from build123d import *

# Parameters (mm, degrees)
SKETCH1_W                  = 20
SKETCH1_H                  = 13.5
BOSS_EXTRUDE1_DEPTH        = 5
F_3_2_3_2_M2_HEAT_SET_D    = 3.2
FILLET2_R                  = 2.5
F_3_2_3_2_DIAMETER_HOLE1_D = 3.2


with BuildPart() as part:
    # Sketch1 → Boss-Extrude1 (new body)
    with BuildSketch(Plane(origin=(0, 0, 0), x_dir=(1, 0, 0), z_dir=(0, 1, 0))):
        Rectangle(SKETCH1_W, SKETCH1_H)
    extrude(amount=BOSS_EXTRUDE1_DEPTH)

    # Ø3.2 (3.2) M2 heat set (through all)
    with Locations(Plane(origin=(0, 5, 0), x_dir=(1, 0, 0), z_dir=(0, 1, 0))):
        with Locations((0, 3.75)):
            Hole(F_3_2_3_2_M2_HEAT_SET_D / 2)

    # Fillet2
    fillet2_edges = [part.edges().sort_by_distance(p)[0] for p in [
        (0, 0, 6.75),
        (0, 5, 6.75),
    ]]
    fillet(fillet2_edges, radius=FILLET2_R - 0.0001)  # a hair under: the kernel refuses the full size

    # Ø3.2 (3.2) Diameter Hole1 (through all)
    with Locations(Plane(origin=(10, 0, 0), x_dir=(0, 0, -1), z_dir=(1, 0, 0))):
        with Locations((-3.75, 2.5)):
            Hole(F_3_2_3_2_DIAMETER_HOLE1_D / 2)


solid = part.part
Can you work these out from the model? Positions are in its coordinate system, mm. Round coordinates to 2 decimals unless told otherwise and drop trailing zeros. Order: outer loops, then holes, each group sorted by start corner. A loop starts at its lowest first (then second) coordinate and runs counter-clockwise, first axis right, second up. Notation, with made-up numbers: (21.5, 2) - (75.5, 2) arc R25 cw to (75.5, 32) - close; hole circle Ø9 at (36, 72). An arc over 180 degrees is marked (long way). Answer in a Markdown table with one row per item.
(1) Suppose I cut it at B-B, the plane z = -3.75. Please give me the cut outline in (x, y), plus the area to 3 significant figures.
From the geometry:
| item | result |
|---|---|
| outline | (-10, 0) - (-1.6, 0) - (-1.6, 5) - (-10, 5) - close; (1.6, 0) - (10, 0) - (10, 5) - (1.6, 5) - close |
| area | 84.0 mm2 |
(2) If we mould it in two halves opening along Y, with no side actions, what happens to faces 1 (the face through (-0.14, 1.89, 5.23)), 2 (the face through (0.35, 2.46, -2.19)), 3 (the face through (0, 0, -1)), 4 (the face through (0.14, 4.248, 6.037))? For each: released by +Y, released by -Y, zero draft, split by the parting line, or undercut.
From the geometry:
| item | result |
|---|---|
| face 1 | undercut |
| face 2 | zero draft |
| face 3 | released by -Y |
| face 4 | released by +Y |
(3) Please list where these lines run through material, in increasing order: L1, parallel to Y at x = 6, z = 3.75; L2, parallel to Z at x = 0, y = 3.8; L3, parallel to Z at x = 0, y = 3.1. Write a range as from..to.
From the geometry:
| item | result |
|---|---|
| L1 | y = 0..0.9, 4.1..5 |
| L2 | z = -6.75..-5.35, -2.15..2.82, 4.68..6.39 |
| L3 | z = -6.75..-5.35, -2.15..2.27, 5.23..6.68 |
(4) For P1, Ø2, axis at x = 3, y = 1, coming from the +Z side, with a flat end and sliding along its axis, tell me the tip position at first contact or that it passes through.
From the geometry:
| item | result |
|---|---|
| P1 | stops at z = 6.7 |
(5) Suppose I cut it at A-A, the plane x = 0. Count the separate pieces of the cut face and the enclosed holes in it, plus the area to 3 significant figures.
From the geometry:
| item | result |
|---|---|
| separate pieces | 2 |
| enclosed holes | 1 |
| area | 40.8 mm2 |
(6) Suppose I cut it at C-C, the plane y = 1.75. Please give me the cut outline in (x, z).
From the geometry:
| item | result |
|---|---|
| outline | (-10, -6.75) - (10, -6.75) - (10, 2.34) - (-10, 2.34) - close; (-10, 5.16) - (10, 5.16) - (10, 6.63) - (-10, 6.63) - close; hole circle Ø3.2 at (0, -3.75) |
